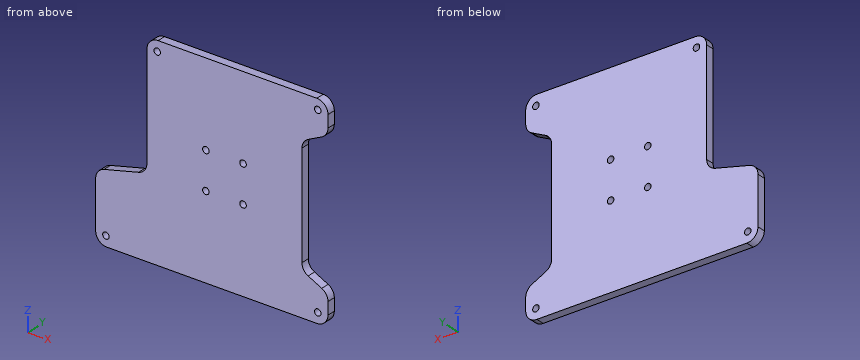
```python
from build123d import *

# Parameters (mm, degrees)
SKETCH1_R           = 1.75
BOSS_EXTRUDE1_DEPTH = 4.5


with BuildPart() as part:
    # Sketch1 → Boss-Extrude1 (new body)
    with BuildSketch(Plane(origin=(0, 0, 0), x_dir=(1, 0, 0), z_dir=(0, 1, 0))):
        with BuildLine():
            Line((-35.7, -55), (49.7, -55))
            ThreePointArc((49.7, -55), (53.942640687, -53.242640687), (55.7, -49))
            Line((55.7, -49), (55.7, -42.377818725))
            ThreePointArc((55.7, -42.377818725), (54.797249664, -39.212689049), (52.36065138, -37))
            Line((52.36065138, -37), (45.03934862, -33.377818725))
            ThreePointArc((45.03934862, -33.377818725), (42.602750336, -31.165129675), (41.7, -28))
            Line((41.7, -28), (41.7, 28))
            ThreePointArc((41.7, 28), (42.602750336, 31.165129675), (45.03934862, 33.377818725))
            Line((45.03934862, 33.377818725), (52.36065138, 37))
            ThreePointArc((52.36065138, 37), (54.797249664, 39.212689049), (55.7, 42.377818725))
            Line((55.7, 42.377818725), (55.7, 49))
            ThreePointArc((55.7, 49), (53.942640687, 53.242640687), (49.7, 55))
            Line((49.7, 55), (-63.3, 55))
            ThreePointArc((-63.3, 55), (-67.542640687, 53.242640687), (-69.3, 49))
            Line((-69.3, 49), (-69.3, 23.31729281))
            ThreePointArc((-69.3, 23.31729281), (-68.03372658, 19.630582533), (-64.769389112, 17.5))
            Line((-64.769389112, 17.5), (-46.230610888, 12.81729281))
            ThreePointArc((-46.230610888, 12.81729281), (-42.96627342, 10.686710277), (-41.7, 7))
            Line((-41.7, 7), (-41.7, -49))
            ThreePointArc((-41.7, -49), (-39.942640687, -53.242640687), (-35.7, -55))
        make_face()
        with Locations(Location((-63.8, 49.5, 0), (0, 0, 270))):
            Circle(SKETCH1_R, mode=Mode.SUBTRACT)
        with Locations(Location((-36.2, -49.5, 0), (0, 0, 270))):
            Circle(SKETCH1_R, mode=Mode.SUBTRACT)
        with Locations(Location((50.2, -49.5, 0), (0, 0, 270))):
            Circle(SKETCH1_R, mode=Mode.SUBTRACT)
        with Locations(Location((50.2, 49.5, 0), (0, 0, 270))):
            Circle(SKETCH1_R, mode=Mode.SUBTRACT)
        with Locations(Location((-10, 10, 0), (0, 0, 270))):
            Circle(SKETCH1_R, mode=Mode.SUBTRACT)
        with Locations(Location((-10, -10, 0), (0, 0, 270))):
            Circle(SKETCH1_R, mode=Mode.SUBTRACT)
        with Locations(Location((10, -10, 0), (0, 0, 270))):
            Circle(SKETCH1_R, mode=Mode.SUBTRACT)
        with Locations(Location((10, 10, 0), (0, 0, 270))):
            Circle(SKETCH1_R, mode=Mode.SUBTRACT)
    extrude(amount=BOSS_EXTRUDE1_DEPTH)


solid = part.part
```
Geometry check sheet. Reference: the model listing, model coordinates, mm. Coordinates: 2 decimals unless noted, no trailing zeros. Loops run counter-clockwise (first coordinate to the right, second up) from the corner with the lowest first, then second, coordinate; pieces in that order, holes last. Notation, with made-up numbers: (32.25, 48) -> (86.25, 48) arc R12 ccw to (86.25, 63) -> close; hole circle Ø8 at (3.25, -27). An arc over 180 degrees is marked (long way). Put each result on its own line as item: value.
1) Cross-section at B-B on y = 2.4. Count the separate pieces of the cut face and the enclosed holes in it, plus the area to 3 significant figures.
Result set:
separate pieces: 1
enclosed holes: 8
area: 10,700 mm^2
2) Cross-section at A-A on x = 10. Record the boundary of the cut face in (y, z).
Result set:
outline: (0, -55) -> (4.5, -55) -> (4.5, -11.75) -> (0, -11.75) -> close; (0, -8.25) -> (4.5, -8.25) -> (4.5, 8.25) -> (0, 8.25) -> close; (0, 11.75) -> (4.5, 11.75) -> (4.5, 55) -> (0, 55) -> close
3) Thickness scan on line 1 (X direction, y = 0.95, z = -49.5); line 2 (X direction, y = 1.85, z = 10); line 3 (Z direction, x = 9, y = 3.9). Record the ranges inside material, lowest first.
Result set:
line 1: x = -69.28 to -65.55, -62.05 to 48.45, 51.95 to 55.68
line 2: x = -41.7 to -11.75, -8.25 to 8.25, 11.75 to 41.7
line 3: z = -55 to -11.44, -8.56 to 8.56, 11.44 to 55
